from build123d import *

# Parameters (mm, degrees)
BOSS_EXTRUDE1_DEPTH = 22.86
SKETCH4_W           = 25.40000152
SKETCH4_H           = 22.86
BOSS_EXTRUDE2_DEPTH = 31.75
BOSS_EXTRUDE3_DEPTH = 22.86
SKETCH6_R           = 2.100001769
CUT_EXTRUDE1_DEPTH  = 22.86


with BuildPart() as part:
    # Sketch3 → Boss-Extrude1 (new body)
    with BuildSketch(Plane.XY.offset(-6.35)):
        with BuildLine():
            Line((-28.0637741, -48), (-2.66377258, -48))
            ThreePointArc((-2.66377258, -48), (32.79872742, -12.5375), (-2.66377258, 22.925))
            Line((-2.66377258, 22.925), (-20.6637745, 22.925))
            Line((-20.6637745, 22.925), (-20.6637745, 4.925))
            Line((-20.6637745, 4.925), (-2.66377258, 4.925))
            ThreePointArc((-2.66377258, 4.925), (14.79872742, -12.5375), (-2.66377258, -30))
            Line((-2.66377258, -30), (-28.0637741, -30))
            Line((-28.0637741, -30), (-28.0637741, -48))
        make_face()
    extrude(amount=-BOSS_EXTRUDE1_DEPTH)

    # Sketch4 → Boss-Extrude2 (add)
    with BuildSketch(Plane.XZ.offset(48)):
        with Locations((-15.36377334, -17.78)):
            Rectangle(SKETCH4_W, SKETCH4_H)
    extrude(amount=BOSS_EXTRUDE2_DEPTH)

    # Sketch5 → Boss-Extrude3 (add)
    with BuildSketch(Plane.XY.offset(-6.35)):
        Polygon((-15.36377334, -79.75), (14.636226604, -79.75), (14.636226604, -97.750000068), (-45.363773284, -97.750000068), (-45.363773284, -79.75), align=None)
    extrude(amount=-BOSS_EXTRUDE3_DEPTH)

    # Sketch6 → Cut-Extrude1 (cut)
    with BuildSketch(Plane.XY.offset(-6.35)):
        with Locations((-35.363773472, -88.750000034)):
            Circle(SKETCH6_R)
        with Locations((4.636226792, -88.750000034)):
            Circle(SKETCH6_R)
    extrude(amount=-CUT_EXTRUDE1_DEPTH, mode=Mode.SUBTRACT)


solid = part.part
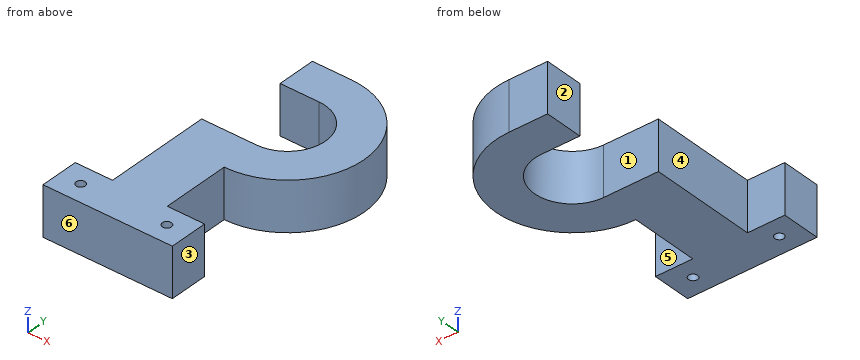
Model file for the job. Use its own axes, mm. Face numbers are marked on the shaded views. A direction names the side the tool comes from. Give positions to 0.01 mm unless a question says otherwise; leave off trailing zeros. Order: outer loops, then holes, each group sorted by start corner. A loop starts at its lowest first (then second) coordinate and runs counter-clockwise, first axis right, second up. Notation, with made-up numbers: (2.5, 78) - (26.5, 78) arc R13 cw to (26.5, 86) - close; hole circle Ø4 at (66, 59). An arc over 180 degrees is marked (long way). One line per item, written item: value.
Item 1: Slice it at D-D (x = -39). List the corners of the cut face in (y, z).
Response values:
outline: (-97.75, -29.21) - (-79.75, -29.21) - (-79.75, -6.35) - (-97.75, -6.35) - close
Item 2: Slice it at B-B (z = -10). Give the number of separate pieces and of enclosed holes in the cut face, then the cut area to 3 significant figures.
Response values:
separate pieces: 1
enclosed holes: 2
area: 4,140 mm2
Item 3: Slice it at C-C (y = -88.75). List the corners of the cut face in (x, z).
Response values:
outline: (-45.36, -29.21) - (-37.46, -29.21) - (-37.46, -6.35) - (-45.36, -6.35) - close; (-33.26, -29.21) - (2.54, -29.21) - (2.54, -6.35) - (-33.26, -6.35) - close; (6.74, -29.21) - (14.64, -29.21) - (14.64, -6.35) - (6.74, -6.35) - close
Item 4: Two-plate mould, pull along Y, no slides. Class the marked faces 4, 5 and 6: released by +Y, released by -Y, zero draft, split by the parting line, or undercut.
Response values:
face 4: zero draft
face 5: undercut
face 6: released by -Y
Item 5: Pin check, flat tips, straight feed: pin 1 Ø7 at (y, z) = (-64, -16) entering from +X; pin 2 Ø12 at (y, z) = (-62, -9.5) entering from -X; pin 3 Ø2 at (x, z) = (18, -23) entering from +Y. Stop position of each tip, or through.
Response values:
pin 1: x = -2.66
pin 2: x = -28.06
pin 3: y = 16.97
Item 6: Wall check: line 1 (X direction, y = -88.75, z = -12.25); line 2 (Y direction, x = -6, z = -11.5) (3 decimals); line 3 (Y direction, x = 13.5, z = -9.75). Give the ranges that are in metal, low to high.
Response values:
line 1: -45.36 to -37.46, -33.26 to 2.54, 6.74 to 14.64
line 2: -97.75 to -30, 4.925 to 22.925
line 3: -97.75 to -79.75, -44.1 to -19.15, -5.93 to 19.03
Item 7: Tool access for the marked faces 1, 2 and 3: list every direction of +Z, -Z, +X, -X, +Y, -Y with a clear straight run to the whole face (end or side of a thin tool).
Response values:
face 1: +Z, -Z, -X
face 2: +Z, -Z, -X, +Y
face 3: +Z, -Z, +X, -Y
Item 8: Slice it at A-A (x = -6). List the corners of the cut face in (y, z) (3 decimals), then the cut area to 3 significant figures.
Response values:
outline: (-97.75, -29.21) - (-30, -29.21) - (-30, -6.35) - (-97.75, -6.35) - close; (4.925, -29.21) - (22.925, -29.21) - (22.925, -6.35) - (4.925, -6.35) - close
area: 1,960 mm2
